Read the model definition and answer for the solid it produces. Units are mm, in the model's axes. Face numbers are marked on the shaded views. A direction names the side the tool comes from. Coordinates: 2 decimals unless noted, no trailing zeros. Write each loop counter-clockwise with the first axis right and the second up, starting at its lowest first coordinate (ties: lowest second). Pieces come first, ordered by that corner, then holes. Notation, with made-up numbers: (24, 30) -> (30, 30) arc R26 cw to (30, 49) -> close; hole circle Ø10 at (33, -6.75). An arc over 180 degrees is marked (long way). Return JSON: item names as keys, results as strings.
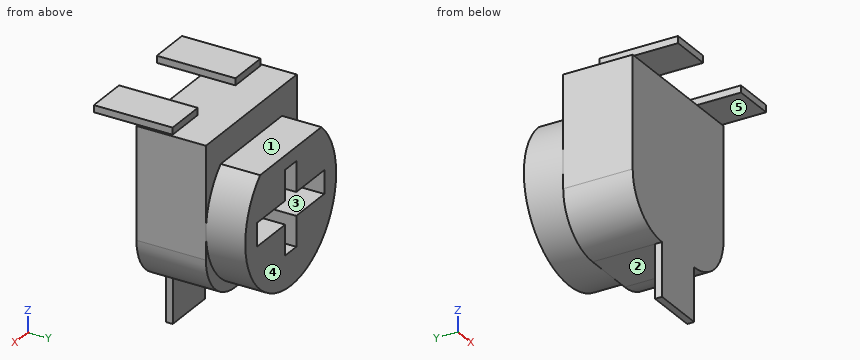
from build123d import *

# Parameters (mm, degrees)
SKETCH_1_W          = 6.5
SKETCH_1_H          = 6.9
EXTRUDE_1_DEPTH     = 3
EXTRUDE_START       = 3
SKETCH_1_3_R        = 3.25
EXTRUDE_2_DEPTH     = 1.7
CUT_EXTRUDE_START   = 3
CUT_EXTRUDE_1_DEPTH = 1.7
FILLET_1_R          = 2.1
SKETCH_2_W          = 1.8
SKETCH_2_H          = 3.4
EXTRUDE_3_DEPTH     = 0.3
SKETCH_3_W          = 2.3
SKETCH_3_H          = 0.3
EXTRUDE_4_DEPTH     = 2.3


with BuildPart() as part:
    # 草图1 → 凸台-拉伸1 (new body)
    with BuildSketch(Plane(origin=(0, 0, 0), x_dir=(1, 0, 0), z_dir=(0, 1, 0))):
        with Locations((0, -0.2)):
            Rectangle(SKETCH_1_W, SKETCH_1_H)
    extrude(amount=EXTRUDE_1_DEPTH)

    # 草图1<3> → 凸台-拉伸2 (add)
    with BuildSketch(Plane(origin=(0, 0, 0), x_dir=(1, 0, 0), z_dir=(0, 1, 0)).offset(EXTRUDE_START)):
        with Locations(Location((0, 0, 0), (0, 0, 90))):
            Circle(SKETCH_1_3_R)
        Polygon((-2.4, -0.5), (-2.4, 0.5), (-0.4, 0.5), (-0.4, 1.8), (0.4, 1.8), (0.4, 0.5), (2.4, 0.5), (2.4, -0.5), (0.4, -0.5), (0.4, -1.8), (-0.4, -1.8), (-0.4, -0.5), align=None, mode=Mode.SUBTRACT)
    extrude(amount=EXTRUDE_2_DEPTH)

    # 草图1<4> → 切除-拉伸1 (cut)
    with BuildSketch(Plane(origin=(0, 0, 0), x_dir=(1, 0, 0), z_dir=(0, 1, 0)).offset(CUT_EXTRUDE_START)):
        with BuildLine():
            Line((2.1914607, -2.4), (-2.1914607, -2.4))
            ThreePointArc((-2.1914607, -2.4), (0, -3.25), (2.1914607, -2.4))
        make_face()
    extrude(amount=CUT_EXTRUDE_1_DEPTH, mode=Mode.SUBTRACT)

    # 圆角1
    fillet_1_edges = [part.edges().sort_by_distance(p)[0] for p in [
        (-3.25, 1.5, -3.25),
        (3.25, 1.5, -3.25),
    ]]
    fillet(fillet_1_edges, radius=FILLET_1_R)

    # 草图2 → 凸台-拉伸3 (add)
    with BuildSketch(Plane.XY.offset(3.65)):
        with Locations((-2.25, -0.2)):
            Rectangle(SKETCH_2_W, SKETCH_2_H)
        with Locations((2.25, -0.2)):
            Rectangle(SKETCH_2_W, SKETCH_2_H)
    extrude(amount=EXTRUDE_3_DEPTH)

    # 草图3 → 凸台-拉伸4 (add)
    with BuildSketch(Plane(origin=(0, 0, -3.25), x_dir=(-1, 0, 0), z_dir=(0, 0, -1))):
        with Locations((0, 0.15)):
            Rectangle(SKETCH_3_W, SKETCH_3_H)
    extrude(amount=EXTRUDE_4_DEPTH)


solid = part.part
1. The part is cut by section A-A (y = -1.5). Determine the outline of the cut face in (x, z).
Taken from the geometry:
{"outline": "(-3.15, 3.65) -> (-1.35, 3.65) -> (-1.35, 3.95) -> (-3.15, 3.95) -> close; (1.35, 3.65) -> (3.15, 3.65) -> (3.15, 3.95) -> (1.35, 3.95) -> close"}
2. Consider L1, parallel to Y at x = 0.5, z = 2.25; L2, parallel to Y at x = -1.5, z = 3.25; L3, parallel to Z at x = 2.5, y = -0.75. Determine where each line is inside the solid, lowest interval first.
Taken from the geometry:
{"L1": "y = 0 to 4.7", "L2": "y = 0 to 3", "L3": "z = 3.65 to 3.95"}
3. The part is cut by section B-B (y = 3.5). Determine the outline of the cut face in (x, z).
Taken from the geometry:
{"outline": "(-2.19, 2.4) arc R3.25 ccw (long way) to (2.19, 2.4) -> close; hole (-2.4, -0.5) -> (-0.4, -0.5) -> (-0.4, -1.8) -> (0.4, -1.8) -> (0.4, -0.5) -> (2.4, -0.5) -> (2.4, 0.5) -> (0.4, 0.5) -> (0.4, 1.8) -> (-0.4, 1.8) -> (-0.4, 0.5) -> (-2.4, 0.5) -> close"}
4. The part is cut by section C-C (z = -1.5). Determine the outline of the cut face in (x, y), then the cut area to 3 significant figures.
Taken from the geometry:
{"outline": "(-3.22, 0) -> (3.22, 0) -> (3.22, 3) -> (2.88, 3) -> (2.88, 4.7) -> (0.4, 4.7) -> (0.4, 3) -> (-0.4, 3) -> (-0.4, 4.7) -> (-2.88, 4.7) -> (-2.88, 3) -> (-3.22, 3) -> close", "area": "27.8 mm2"}
5. A tool of negligible diameter and unlimited length cuts with its end or side. For the marked faces 1, 2, 3, 4 and 5, from which of +Z, -Z, +X, -X, +Y, -Y can it reach the whole face along a straight path? Write none if from no direction.
Taken from the geometry:
{"face 1": "+Z, +X, -X, +Y", "face 2": "-Z, +X, -X, +Y", "face 3": "+Y", "face 4": "+Z, -Z, +X, -X, +Y", "face 5": "-Z, +X, -X, -Y"}
6. The part is cut by section D-D (x = -1). Determine the outline of the cut face in (y, z), then the cut area to 3 significant figures.
Taken from the geometry:
{"outline": "(0, -5.55) -> (0.3, -5.55) -> (0.3, -3.25) -> (3, -3.25) -> (3, -3.09) -> (4.7, -3.09) -> (4.7, -0.5) -> (3, -0.5) -> (3, 0.5) -> (4.7, 0.5) -> (4.7, 2.4) -> (3, 2.4) -> (3, 3.65) -> (0, 3.65) -> close", "area": "29.0 mm2"}
7. Flat-ended cylindrical pins translate along their axes: pin 1 Ø0.6 at (y, z) = (3.5, 1.5) entering from +X; pin 2 Ø0.8 at (x, y) = (-1, 3.5) entering from +Z; pin 3 Ø0.6 at (x, y) = (0, 4) entering from -Z. Find the tip coordinate at first contact, or state that the pin passes through.
Taken from the geometry:
{"pin 1": "stops at x = 3.02", "pin 2": "stops at z = 2.4", "pin 3": "stops at z = -3.25"}
